from build123d import *

# Parameters (mm, degrees)
ESQUISSE1_W             = 10
ESQUISSE1_H             = 20
BOSS_EXTRU_1_DEPTH      = 11
BOSS_EXTRU_1_2_DEPTH    = 11
ESQUISSE3_W             = 40
ESQUISSE3_H             = 20
BOSS_EXTRU_2_DEPTH      = 12
ENL_V_MAT_EXTRU_1_REACH = 25
ESQUISSE4_R             = 3.2
ESQUISSE1_3_R           = 2.75
ENL_V_MAT_EXTRU_3_DEPTH = 15
ESQUISSE1_4_R           = 3.5
ESQUISSE1_4_R_2         = 2.75
ENL_V_MAT_EXTRU_4_DEPTH = 1
CHANFREIN1_SIZE         = 3
CONG_1_R                = 3
ESQUISSE6_W             = 10.5
ESQUISSE6_H             = 20
ENL_V_MAT_EXTRU_5_DEPTH = 5


with BuildPart() as part:
    # Esquisse1 → Boss.-Extru.1 (new body)
    with BuildSketch(Plane(origin=(0, 0, 0), x_dir=(1, 0, 0), z_dir=(0, 1, 0))):
        with Locations((-15, 0)):
            Rectangle(ESQUISSE1_W, ESQUISSE1_H)
    extrude(amount=BOSS_EXTRU_1_DEPTH)



with BuildPart() as body_2:
    # Esquisse1 → Boss.-Extru.1 2 (new body)
    with BuildSketch(Plane(origin=(0, 0, 0), x_dir=(1, 0, 0), z_dir=(0, 1, 0))):
        with Locations((15, 0)):
            Rectangle(ESQUISSE1_W, ESQUISSE1_H)
    extrude(amount=BOSS_EXTRU_1_2_DEPTH)


with BuildPart() as part_1:
    add(part.part)

    add(body_2.part)  # Boss.-Extru.2 merges body 2
    # Esquisse3 → Boss.-Extru.2 (add)
    with BuildSketch(Plane(origin=(0, 11, 0), x_dir=(1, 0, 0), z_dir=(0, 1, 0))):
        Rectangle(ESQUISSE3_W, ESQUISSE3_H)
    extrude(amount=BOSS_EXTRU_2_DEPTH)

    # Esquisse4 → Enl_v. mat.-Extru.1 (cut, up to next)
    with BuildSketch(Plane(origin=(0, 23, 0), x_dir=(1, 0, 0), z_dir=(0, 1, 0)), mode=Mode.PRIVATE) as enl_v_mat_extru_1_sk1:
        Circle(ESQUISSE4_R)
    enl_v_mat_extru_1_tool1 = extrude(enl_v_mat_extru_1_sk1.sketch, amount=-ENL_V_MAT_EXTRU_1_REACH, mode=Mode.PRIVATE) & part_1.part
    add(enl_v_mat_extru_1_tool1.solids().sort_by_distance((0, 23, 0))[0], mode=Mode.SUBTRACT)

    # Esquisse1_3 → Enl_v. mat.-Extru.3 (cut)
    with BuildSketch(Plane(origin=(0, 0, 0), x_dir=(1, 0, 0), z_dir=(0, 1, 0))):
        with Locations((-15, 0)):
            Circle(ESQUISSE1_3_R)
        with Locations((15, 0)):
            Circle(ESQUISSE1_3_R)
    extrude(amount=ENL_V_MAT_EXTRU_3_DEPTH, mode=Mode.SUBTRACT)

    # Esquisse1_4 → Enl_v. mat.-Extru.4 (cut)
    with BuildSketch(Plane(origin=(0, 0, 0), x_dir=(1, 0, 0), z_dir=(0, 1, 0))):
        with Locations((-15, 0)):
            Circle(ESQUISSE1_4_R)
        with Locations((-15, 0)):
            Circle(ESQUISSE1_4_R_2, mode=Mode.SUBTRACT)
        with Locations((15, 0)):
            Circle(ESQUISSE1_4_R)
        with Locations((15, 0)):
            Circle(ESQUISSE1_4_R_2, mode=Mode.SUBTRACT)
    extrude(amount=ENL_V_MAT_EXTRU_4_DEPTH, mode=Mode.SUBTRACT)

    # Chanfrein1
    chanfrein1_edges = [part_1.edges().sort_by_distance(p)[0] for p in [
        (20, 11.5, 10),
        (20, 11.5, -10),
        (10, 5.5, -10),
        (10, 5.5, 10),
        (-20, 11.5, 10),
        (-20, 11.5, -10),
        (-10, 5.5, -10),
        (-10, 5.5, 10),
    ]]
    chamfer(chanfrein1_edges, length=CHANFREIN1_SIZE)

    # Cong_1
    cong_1_edges = [part_1.edges().sort_by_distance(p)[0] for p in [
        (-20, 11.5, -7),
        (10, 5.5, 7),
        (10, 5.5, -7),
        (-17, 11.5, -10),
        (-13, 5.5, -10),
        (17, 11.5, -10),
        (13, 5.5, -10),
        (20, 11.5, 7),
        (20, 11.5, -7),
        (-17, 11.5, 10),
        (17, 11.5, 10),
        (-13, 5.5, 10),
        (13, 5.5, 10),
        (-10, 5.5, 7),
        (-10, 5.5, -7),
        (-20, 11.5, 7),
    ]]
    fillet(cong_1_edges, radius=CONG_1_R)

    # Esquisse6 → Enl_v. mat.-Extru.5 (cut)
    with BuildSketch(Plane(origin=(0, 14.5, 0), x_dir=(-1, 0, 0), z_dir=(0, -1, 0))):
        Rectangle(ESQUISSE6_W, ESQUISSE6_H)
    extrude(amount=-ENL_V_MAT_EXTRU_5_DEPTH, mode=Mode.SUBTRACT)


solid = part_1.part
The listing builds one solid part. Answer for the finished solid, in the listing's coordinates (mm). A direction names the side the tool comes from. Round coordinates to 2 decimals unless told otherwise and drop trailing zeros. Write each loop counter-clockwise with the first axis right and the second up, starting at its lowest first coordinate (ties: lowest second). Pieces come first, ordered by that corner, then holes. Notation, with made-up numbers: (-12, -40) - (3, -40) arc R27 ccw to (3, -8) - close; hole circle Ø8 at (80, 77.25). An arc over 180 degrees is marked (long way). Use one line per item in the form item = value. Start each with the question number.
Item 1: A cutting plane is placed at C-C (x = 0). Write down the section's boundary in (y, z).
Item 2: A cutting plane is placed at D-D (x = 13). Write down the section's boundary in (y, z).
Item 3: A cutting plane is placed at A-A (y = 15.75). Write down the section's boundary in (x, z), plus the area to 3 significant figures.
Item 4: Flat-ended cylindrical pins translate along their axes: pin 1 Ø3 at (x, z) = (15.5, -1) entering from -Y; pin 2 Ø10 at (x, z) = (0, 0) entering from -Y. Find the tip coordinate at first contact, or state that the pin passes through.
Item 5: Determine the mould class of faces 1 (the cylindrical face through (13.079, 5.577, -9.765)), 2 (the flat face through (0, 14, 10)), 3 (the cylindrical face through (19.78, 11.34, -6.89)) for opening direction X: +X half, -X half, draft (parallel to the pull), parting line (faces both ways), or undercut.
Item 6: Find the intervals of material crossed by line 1 (X direction, y = 0.7, z = 0); line 2 (Z direction, x = 0, y = 20.6); line 3 (Z direction, x = 15, y = 10.75), in increasing order. Write a range as [from, to].
Item 7: A cutting plane is placed at B-B (z = -4.75). Write down the section's boundary in (x, y).
Item 8: A tool of negligible diameter and unlimited length cuts with its end or side. For faces 4 (the flat face through (10, 5, 0)), 5 (the flat face through (-5.25, 17, 0)), 6 (the cylindrical face through (10.22, 5.58, 6.89)), 7 (the flat face through (11, 5, -8)), 8 (the flat face through (-15, 15, 0)), from which of +Z, -Z, +X, -X, +Y, -Y can it reach the whole face along a straight path? Write none if from no direction.
The answers:
q1.outline = (11, -10) - (14.5, -10) - (14.5, -3.2) - (11, -3.2) - close; (11, 3.2) - (14.5, 3.2) - (14.5, 10) - (11, 10) - close; (19.5, -10) - (23, -10) - (23, -3.2) - (19.5, -3.2) - close; (19.5, 3.2) - (23, 3.2) - (23, 10) - (19.5, 10) - close
q2.outline = (0, -9.73) - (11, -9.73) - (11, -10) - (23, -10) - (23, 10) - (11, 10) - (11, 9.73) - (0, 9.73) - (0, 2.87) - (1, 2.87) - (1, 1.89) - (15, 1.89) - (15, -1.89) - (1, -1.89) - (1, -2.87) - (0, -2.87) - close
q3.outline = (-20, -5.76) arc R3 ccw to (-19.12, -7.88) - (-17.88, -9.12) arc R3 ccw to (-15.76, -10) - (-5.25, -10) - (-5.25, 10) - (-15.76, 10) arc R3 ccw to (-17.88, 9.12) - (-19.12, 7.88) arc R3 ccw to (-20, 5.76) - close; (5.25, -10) - (15.76, -10) arc R3 ccw to (17.88, -9.12) - (19.12, -7.88) arc R3 ccw to (20, -5.76) - (20, 5.76) arc R3 ccw to (19.12, 7.88) - (17.88, 9.12) arc R3 ccw to (15.76, 10) - (5.25, 10) - close
q3.area = 570 mm^2
q4.pin_1 = 15
q4.pin_2 = 11
q5.face_1 = undercut
q5.face_2 = draft
q5.face_3 = +X half
q6.line_1 = [-20, -18.5], [-11.5, -10], [10, 11.5], [18.5, 20]
q6.line_2 = [-10, -3.2], [3.2, 10]
q6.line_3 = [-10, -2.75], [2.75, 10]
q7.outline = (-20, 0) - (-10, 0) - (-10, 11) - (10, 11) - (10, 0) - (20, 0) - (20, 23) - (-20, 23) - close; hole (-5.25, 14.5) - (5.25, 14.5) - (5.25, 19.5) - (-5.25, 19.5) - close
q8.face_4 = +Z, -Z, -Y
q8.face_5 = +Z, -Z
q8.face_6 = +Z, -Y
q8.face_7 = -Z, -Y
q8.face_8 = -Y
